Model file for the job. Use its own axes, mm. Face numbers are marked on the shaded views. A direction names the side the tool comes from. Round coordinates to 2 decimals unless told otherwise and drop trailing zeros. Loops run counter-clockwise (first coordinate to the right, second up) from the corner with the lowest first, then second, coordinate; pieces in that order, holes last. Notation, with made-up numbers: (50.5, 12) -> (70.5, 12) arc R21 cw to (70.5, 31) -> close; hole circle Ø6 at (-37, 85). An arc over 180 degrees is marked (long way). Use a Markdown table: item, result. Add a question column.
```python
from build123d import *

# Parameters (mm, degrees)
F0_W     = 141.6642213652
F0_H     = 10
F1_DEPTH = 20
F2_R     = 10
F3_DEPTH = 90
F4_W     = 141.6642213652
F4_H     = 20
F5_DEPTH = 10
F6_R     = 9.9999


# Not quite as in the source:
# - a fillet or chamfer is up to 0.001 mm smaller than in the source, because OpenCascade refuses the exact size


with BuildPart() as f1:
    # F0 (on Front) → F1 (new body)
    with BuildSketch(Plane.XZ):
        with Locations((-0.8321106826, -5)):
            Rectangle(F0_W, F0_H)
    extrude(amount=F1_DEPTH)

    # F2 (on face) → F3 (join)
    with BuildSketch(Plane.XY):
        with Locations((-61.6642213652, -10)):
            Circle(F2_R)
        with Locations((60, -10)):
            Circle(F2_R)
    extrude(amount=F3_DEPTH)

    # F4 (on face) → F5 (join)
    with BuildSketch(Plane.XY.offset(90)):
        with Locations((-0.8321106826, -10)):
            Rectangle(F4_W, F4_H)
    extrude(amount=F5_DEPTH)

    # F6 (radius 10 in the source; OpenCascade refuses exactly that, so slightly less here)
    f6_edges = [f1.edges().sort_by_distance(p)[0] for p in [
        (-71.664221, -20, -5),
        (-71.664221, 0, -5),
        (-71.664221, -20, 95),
        (-71.664221, 0, 95),
        (70, 0, 95),
        (70, -20, 95),
        (70, 0, -5),
        (70, -20, -5),
    ]]
    fillet(f6_edges, radius=F6_R)


solid = f1.part
```
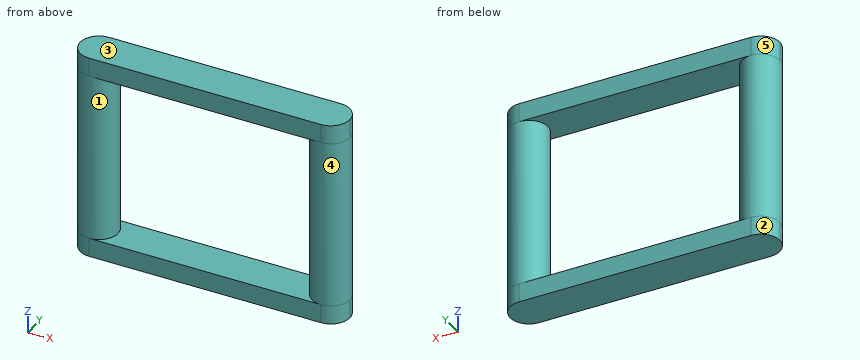
1) Wall check: probe 1 along Z at (x, y) = (4, -15.75); probe 2 along X at (y, z) = (-13, 15); probe 3 along X at (y, z) = (-12.25, 40.5). Give the ranges that are in metal, low to high. Write a range as from..to.
2) Pull direction X, two halves, no side cores. Call the marked faces 1, 2 and 3: +X half, -X half, draft (parallel to the pull), parting line (faces both ways), or undercut.
3) Tool access for the marked faces 4 and 5: list every direction of +Z, -Z, +X, -X, +Y, -Y with a clear straight run to the whole face (end or side of a thin tool).
4) Cut at C-C on z = 31. Write the cut outline in (x, y).
5) Pin check, flat tips, straight feed: pin 1 Ø2 at (y, z) = (-18, 39) entering from +X; pin 2 Ø12 at (y, z) = (-6.5, 51) entering from -X; pin 3 Ø8 at (y, z) = (-17.5, 76) entering from +X; pin 4 Ø2 at (x, z) = (-54, 58.5) entering from +Y. Stop position of each tip, or through.
6) Cut at A-A on x = 35. Write the cut outline in (y, z), and give its area (3 significant figures).
Established:
| question | item | result |
|---|---|---|
| 1 | probe 1 | z = -10..0, 90..100 |
| 1 | probe 2 | x = -71.2..-52.12, 50.46..69.54 |
| 1 | probe 3 | x = -71.41..-51.92, 50.26..69.74 |
| 2 | face 1 | undercut |
| 2 | face 2 | -X half |
| 2 | face 3 | draft |
| 3 | face 4 | none |
| 3 | face 5 | +Z, -Z, -X, +Y |
| 4 | outline | circle Ø20 at (-61.66, -10); circle Ø20 at (60, -10) |
| 5 | pin 1 | stops at x = 67.14 |
| 5 | pin 2 | stops at x = -71.66 |
| 5 | pin 3 | stops at x = 69.37 |
| 5 | pin 4 | stops at y = -2.54 |
| 6 | outline | (-20, -10) -> (0, -10) -> (0, 0) -> (-20, 0) -> close; (-20, 90) -> (0, 90) -> (0, 100) -> (-20, 100) -> close |
| 6 | area | 400 mm^2 |
